from build123d import *

# Parameters (mm, degrees)
SKETCH1_W           = 32
SKETCH1_H           = 53
SKETCH1_W_2         = 22
SKETCH1_H_2         = 42
BOSS_EXTRUDE1_DEPTH = 20
SKETCH2_W           = 5
SKETCH2_H           = 20
BOSS_EXTRUDE2_DEPTH = 30
SKETCH3_R           = 2.75
SKETCH3_R_2         = 1.6
CUT_EXTRUDE1_DEPTH  = 3
SKETCH3_2_R         = 1.6
CUT_EXTRUDE2_DEPTH  = 63.69968102
SKETCH4_R           = 1.5
CUT_EXTRUDE3_DEPTH  = 59.806887352
FILLET1_R           = 5
FILLET2_R           = 2


with BuildPart() as part:
    # Sketch1 → Boss-Extrude1 (new body)
    with BuildSketch(Plane.XY):
        Rectangle(SKETCH1_W, SKETCH1_H)
        Rectangle(SKETCH1_W_2, SKETCH1_H_2, mode=Mode.SUBTRACT)
    extrude(amount=BOSS_EXTRUDE1_DEPTH)

    # Sketch2 → Boss-Extrude2 (add)
    with BuildSketch(Plane.XY.offset(20)):
        with Locations((-13.5, -11.5)):
            Rectangle(SKETCH2_W, SKETCH2_H)
    extrude(amount=BOSS_EXTRUDE2_DEPTH)

    # Sketch3 → Cut-Extrude1 (cut)
    # profile 1 of 2: a face of its own
    with BuildSketch(Plane(origin=(-11, 0, 0), x_dir=(0, 0, -1), z_dir=(1, 0, 0))):
        with Locations((-42, -11.5)):
            Circle(SKETCH3_R)
        with Locations((-42, -11.5)):
            Circle(SKETCH3_R_2, mode=Mode.SUBTRACT)
    # profile 2 of 2: a face of its own
    with BuildSketch(Plane(origin=(-11, 0, 0), x_dir=(0, 0, -1), z_dir=(1, 0, 0))):
        with Locations((-28, -11.5)):
            Circle(SKETCH3_R)
        with Locations((-28, -11.5)):
            Circle(SKETCH3_R_2, mode=Mode.SUBTRACT)
    extrude(amount=-CUT_EXTRUDE1_DEPTH, mode=Mode.SUBTRACT)

    # Sketch3<2> → Cut-Extrude2 (cut, through all)
    with BuildSketch(Plane(origin=(-11, 0, 0), x_dir=(0, 0, -1), z_dir=(1, 0, 0))):
        with Locations((-42, -11.5)):
            Circle(SKETCH3_2_R)
        with Locations((-28, -11.5)):
            Circle(SKETCH3_2_R)
    extrude(amount=-CUT_EXTRUDE2_DEPTH, mode=Mode.SUBTRACT)

    # Sketch4 → Cut-Extrude3 (cut, through all)
    with BuildSketch(Plane(origin=(0, 0, 0), x_dir=(-1, 0, 0), z_dir=(0, 0, -1))):
        with Locations((-5.1, -23.9)):
            Circle(SKETCH4_R)
        with Locations((5.1, -23.9)):
            Circle(SKETCH4_R)
        with Locations((-5.1, 23.9)):
            Circle(SKETCH4_R)
        with Locations((5.1, 23.9)):
            Circle(SKETCH4_R)
    extrude(amount=-CUT_EXTRUDE3_DEPTH, mode=Mode.SUBTRACT)

    # Fillet1
    fillet1_edges = [part.edges().sort_by_distance(p)[0] for p in [
        (16, -26.5, 10),
        (-16, -26.5, 10),
        (-16, 26.5, 10),
        (16, 26.5, 10),
    ]]
    fillet(fillet1_edges, radius=FILLET1_R)

    # Fillet2
    fillet2_edges = [part.edges().sort_by_distance(p)[0] for p in [
        (-16, -1.5, 35),
        (-16, -21.5, 35),
        (-11, -1.5, 35),
        (-11, -21.5, 35),
    ]]
    fillet(fillet2_edges, radius=FILLET2_R)


solid = part.part
Build history of the part. All positions in model axes, mm. A direction names the side the tool comes from. Coordinates: 2 decimals unless noted, no trailing zeros. Write each loop counter-clockwise with the first axis right and the second up, starting at its lowest first coordinate (ties: lowest second). Pieces come first, ordered by that corner, then holes. Notation, with made-up numbers: (39.25, -8) -> (81.25, -8) arc R19 cw to (81.25, 25) -> close; hole circle Ø7 at (85, 24). An arc over 180 degrees is marked (long way). Use CSV: the item, a comma, the result in double quotes. Start each with the question number.
Q1. Pull direction Z, two halves, no side cores. Call faces 6 (the cylindrical face through (-14.99, -12.47, 29.27)), 7 (the flat face through (-14, -11, 50)), 8 (the cylindrical face through (-15.43, -20.9, 35.21)): released by +Z, released by -Z, zero draft, split by the parting line, or undercut.
Q2. Cut at B-B, the plane z = 42. List the corners of the cut face in (x, y), then the cut area to 3 significant figures.
Q3. Cut at A-A, the plane y = -11.5. List the corners of the cut face in (x, z).
Q4. 3-axis set-ups, long thin cutter, end or side, ignore diameter. For faces 1 (the flat face through (14, 0, 0)), 2 (the cylindrical face through (-14.57, 25, 10.14)), 3 (the flat face through (0, 21, 10)), 4 (the cylindrical face through (-15.43, -2.1, 35.21)), 5 (the cylindrical face through (-12.479, -11.379, 44.747)): which of +Z, -Z, +X, -X, +Y, -Y reach the whole face in a straight line?
Q5. Cut at C-C, the plane x = 2.5. List the corners of the cut face in (y, z), then the cut area to 3 significant figures.
Q6. Drill centre lines: probe 1 along Y at (x, z) = (-5.1, 10.25); probe 2 along X at (y, z) = (-7, 11); probe 3 along Y at (x, z) = (10, 11.5). Where is each one in solid material? Low to high.
Q7. Cut at D-D, the plane y = 13.5. List the corners of the cut face in (x, z), then the cut area to 3 significant figures.
Q8. Flat gauge pins, fed straight in: pin 1 Ø5 at (x, y) = (-5.1, -23.9) entering from +Z; pin 2 Ø0.8 at (x, z) = (-13.5, 35) entering from +Y; pin 3 Ø4.5 at (y, z) = (-10.5, 27) entering from +X. Where does each tip first touch, or does it go through?
Checked values:
1,face 6,"undercut"
1,face 7,"released by +Z"
1,face 8,"zero draft"
2,outline,"(-16, -19.5) arc R2 ccw to (-14, -21.5) -> (-13, -21.5) arc R2 ccw to (-11, -19.5) -> (-11, -14.25) -> (-14, -14.25) -> (-14, -13.1) -> (-16, -13.1) -> close; (-16, -9.9) -> (-14, -9.9) -> (-14, -8.75) -> (-11, -8.75) -> (-11, -3.5) arc R2 ccw to (-13, -1.5) -> (-14, -1.5) arc R2 ccw to (-16, -3.5) -> close"
2,area,"73.7 mm²"
3,outline,"(-16, 0) -> (-11, 0) -> (-11, 25.25) -> (-14, 25.25) -> (-14, 26.4) -> (-16, 26.4) -> close; (-16, 29.6) -> (-14, 29.6) -> (-14, 30.75) -> (-11, 30.75) -> (-11, 39.25) -> (-14, 39.25) -> (-14, 40.4) -> (-16, 40.4) -> close; (-16, 43.6) -> (-14, 43.6) -> (-14, 44.75) -> (-11, 44.75) -> (-11, 50) -> (-16, 50) -> close; (11, 0) -> (16, 0) -> (16, 20) -> (11, 20) -> close"
4,face 1,"-Z, +X, -X, +Y, -Y"
4,face 2,"+Z, -Z, -X, +Y"
4,face 3,"+Z, -Z"
4,face 4,"+Z, -X, +Y"
4,face 5,"+X"
5,outline,"(-26.5, 0) -> (-21, 0) -> (-21, 20) -> (-26.5, 20) -> close; (21, 0) -> (26.5, 0) -> (26.5, 20) -> (21, 20) -> close"
5,area,"220 mm²"
6,probe 1,"y = -26.5 to -25.4, -22.4 to -21, 21 to 22.4, 25.4 to 26.5"
6,probe 2,"x = -16 to -11, 11 to 16"
6,probe 3,"y = -26.5 to -21, 21 to 26.5"
7,outline,"(-16, 0) -> (-11, 0) -> (-11, 20) -> (-16, 20) -> close; (11, 0) -> (16, 0) -> (16, 20) -> (11, 20) -> close"
7,area,"200 mm²"
8,pin 1,"stops at z = 20"
8,pin 2,"stops at y = -1.5"
8,pin 3,"stops at x = -11"
